from build123d import *

# Parameters (mm, degrees)
BOSS_EXTRUDE1_DEPTH = 6.35
CUT_EXTRUDE1_DEPTH  = 212.560806862
SKETCH4_W           = 6.35
SKETCH4_H           = 63.5
SKETCH4_H_2         = 81.28
BOSS_EXTRUDE3_DEPTH = 6.35
SKETCH5_R           = 1.4732
CUT_EXTRUDE2_DEPTH  = 216.806597443
SKETCH6_R           = 3.175
SKETCH6_R_2         = 1.4732
CUT_EXTRUDE3_DEPTH  = 216.806597443
CUT_EXTRUDE4_REACH  = 217.807
SKETCH7_R           = 3.175
SKETCH8_R           = 1.4605
CUT_EXTRUDE5_DEPTH  = 216.806597443


with BuildPart() as part:
    # Sketch1 → Boss-Extrude1 (new body)
    with BuildSketch(Plane(origin=(0, 0, 0), x_dir=(0, 0, -1), z_dir=(1, 0, 0))):
        Polygon((0, 0), (139.7, 0), (139.7, 158.75), (76.2, 158.75), (76.2, 152.4), (0, 152.4), (-50.8, 152.4), (-50.8, 158.75), (-107.95, 158.75), (-107.95, 107.95), (0, 107.95), align=None)
    extrude(amount=BOSS_EXTRUDE1_DEPTH)

    # Sketch2 → Cut-Extrude1 (cut, through all)
    with BuildSketch(Plane.ZY):
        Polygon((0, 17.5768), (-3.96875, 17.5768), (-3.96875, 15.875), (-6.35, 15.875), (-6.35, 17.5768), (-12.7, 17.5768), (-12.7, 20.5232), (-6.35, 20.5232), (-6.35, 22.225), (-3.96875, 22.225), (-3.96875, 20.5232), (0, 20.5232), align=None)
        Polygon((-139.7, 17.5768), (-139.7, 20.5232), (-135.73125, 20.5232), (-135.73125, 22.225), (-133.35, 22.225), (-133.35, 20.5232), (-127, 20.5232), (-127, 17.5768), (-133.35, 17.5768), (-133.35, 15.875), (-135.73125, 15.875), (-135.73125, 17.5768), align=None)
        Polygon((-133.35, 136.525), (-133.35, 134.8232), (-127, 134.8232), (-127, 131.8768), (-133.35, 131.8768), (-133.35, 130.175), (-135.73125, 130.175), (-135.73125, 131.8768), (-139.7, 131.8768), (-139.7, 134.8232), (-135.73125, 134.8232), (-135.73125, 136.525), align=None)
    extrude(amount=-CUT_EXTRUDE1_DEPTH, mode=Mode.SUBTRACT)

    # Sketch4 → Boss-Extrude3 (add)
    with BuildSketch(Plane.ZY):
        with Locations((3.175, 76.2)):
            Rectangle(SKETCH4_W, SKETCH4_H)
        with Locations((-142.875, 76.2)):
            Rectangle(SKETCH4_W, SKETCH4_H_2)
    extrude(amount=-BOSS_EXTRUDE3_DEPTH)

    # Sketch5 → Cut-Extrude2 (cut, through all)
    with BuildSketch(Plane.ZY):
        with Locations(Location((3.175, 76.2, 0), (0, 0, 180))):
            Circle(SKETCH5_R)
        with Locations((-142.875, 41.91)):
            Circle(SKETCH5_R)
        with Locations(Location((-142.875, 110.49, 0), (0, 0, 180))):
            Circle(SKETCH5_R)
    extrude(amount=-CUT_EXTRUDE2_DEPTH, mode=Mode.SUBTRACT)

    # Sketch6 → Cut-Extrude3 (cut, through all)
    with BuildSketch(Plane.ZY):
        with Locations((-92.71, 133.35)):
            Circle(SKETCH6_R)
        with Locations((-107.95, 155.575)):
            Circle(SKETCH6_R_2)
        with Locations((-73.914, 136.503809764)):
            Circle(SKETCH6_R)
        with Locations((82.55, 155.575)):
            Circle(SKETCH6_R_2)
        with Locations((77.227381395, 133.35)):
            Circle(SKETCH6_R)
        with Locations((53.096, 136.503809756)):
            Circle(SKETCH6_R)
        with Locations((-10.409000001, 121.89880976)):
            Circle(SKETCH6_R)
        with Locations((-10.408999999, 148.476804796)):
            Circle(SKETCH6_R)
        Polygon((-42.9641, 152.4), (-45.9105, 152.4), (-45.9105, 148.59), (-47.7393, 148.59), (-47.7393, 146.05), (-45.9105, 146.05), (-45.9105, 139.7), (-42.9641, 139.7), (-42.9641, 146.05), (-41.1353, 146.05), (-41.1353, 148.59), (-42.9641, 148.59), align=None)
        Polygon((20.5359, 152.4), (17.5895, 152.4), (17.5895, 148.59), (15.7607, 148.59), (15.7607, 146.05), (17.5895, 146.05), (17.5895, 139.7), (20.5359, 139.7), (20.5359, 146.05), (22.3647, 146.05), (22.3647, 148.59), (20.5359, 148.59), align=None)
    extrude(amount=-CUT_EXTRUDE3_DEPTH, mode=Mode.SUBTRACT)

    # Sketch7 → Cut-Extrude4 (cut, up to next)
    with BuildSketch(Plane(origin=(6.35, 0, 0), x_dir=(0, 0, -1), z_dir=(1, 0, 0)), mode=Mode.PRIVATE) as cut_extrude4_sk1:
        with Locations((141.119403898, 94.059701015)):
            Circle(SKETCH7_R)
    cut_extrude4_tool1 = extrude(cut_extrude4_sk1.sketch, amount=-CUT_EXTRUDE4_REACH, mode=Mode.PRIVATE) & part.part
    add(cut_extrude4_tool1.solids().sort_by_distance((6.35, 94.059701, -141.119404))[0], mode=Mode.SUBTRACT)

    # Sketch8 → Cut-Extrude5 (cut, through all)
    with BuildSketch(Plane.ZY):
        with Locations((31.75, 114.3)):
            Circle(SKETCH8_R)
        with Locations((31.75, 139.7)):
            Circle(SKETCH8_R)
    extrude(amount=-CUT_EXTRUDE5_DEPTH, mode=Mode.SUBTRACT)


solid = part.part
Can you work these out from the model? Positions are in its coordinate system, mm. A direction names the side the tool comes from. Give positions to 0.01 mm unless a question says otherwise; leave off trailing zeros. Order: outer loops, then holes, each group sorted by start corner. A loop starts at its lowest first (then second) coordinate and runs counter-clockwise, first axis right, second up. Notation, with made-up numbers: M 35.25,18.25 L 40.25,18.25 A18 cw 40.25,46.25 Z; hole C -35.5,14.25 d8. An arc over 180 degrees is marked long. One line per item, written item: value.
Item 1: If we section it at B-B on z = 60: Write out the boundary of the cut face in (x, y), and give its area (3 significant figures).
Verdict:
outline: M 0,107.95 L 6.35,107.95 L 6.35,158.75 L 0,158.75 Z
area: 323 mm2
Item 2: For faces 1 (the face through (3, 17.577, -9)), 2 (the face through (3, 17.577, -130)), 3 (the face through (3, 44.45, 3)), 4 (the face through (3, 143, 20.536)), 5 (the face through (3, 124, -139.7)), which set-ups out of +Z, -Z, +X, -X, +Y, -Y let a thin tool reach every point of the face, with its end or its side?
Verdict:
face 1: +Z, +X, -X
face 2: -Z, +X, -X
face 3: +Z, +X, -X, -Y
face 4: +X, -X, +Y
face 5: -Z, +X, -X, +Y
Item 3: Please list where these lines run through material, in increasing order: line 1 (Y direction, x = 1.75, z = 31.75); line 2 (Z direction, x = 3.75, y = 142); line 3 (Z direction, x = 3.25, y = 16).
Verdict:
line 1: 107.95 to 112.84, 115.76 to 138.24, 141.16 to 152.4
line 2: -139.7 to -45.91, -42.96 to 17.59, 20.54 to 107.95
line 3: -139.7 to -135.73, -133.35 to -6.35, -3.97 to 0
Item 4: For pin 1 (1.4 mm diameter, centred on x = 3.5, y = 16.5, fed in from -Z); pin 2 (1.5 mm diameter, centred on x = 2, y = 133, fed in from -Z), each with a flat end and sliding along its axis, tell me the tip position at first contact or that it passes through.
Verdict:
pin 1: z = -139.7
pin 2: z = -127
Item 5: If we section it at C-C on z = -53: Write out the boundary of the cut face in (x, y).
Verdict:
outline: M 0,0 L 6.35,0 L 6.35,152.4 L 0,152.4 Z
Item 6: If we mould it in two halves opening along Y, with no side actions, what happens to faces 6 (the face through (3, 9, 0)), 7 (the face through (3.131, 145.377, -11.097)), 8 (the face through (3, 152.4, 35))? For each: pulls with the +Y half, pulls with the -Y half, needs draft (parallel to the pull), parting line crosses it, or undercut.
Verdict:
face 6: needs draft
face 7: undercut
face 8: pulls with the +Y half
Item 7: If we section it at A-A on z = -92.71: Write out the boundary of the cut face in (x, y) (3 decimals).
Verdict:
outline: M 0,0 L 6.35,0 L 6.35,130.175 L 0,130.175 Z; M 0,136.525 L 6.35,136.525 L 6.35,158.75 L 0,158.75 Z
